Could you check a few things on this model? Use its own coordinates, in mm. Face numbers are marked on the shaded views. Coordinates: 2 decimals unless noted, no trailing zeros. Order: outer loops, then holes, each group sorted by start corner. A loop starts at its lowest first (then second) coordinate and runs counter-clockwise, first axis right, second up. Notation, with made-up numbers: M -22,29 L -3,29 A32 cw -3,65 Z; hole C 65,-39.75 d1. An arc over 180 degrees is marked long. Put each result on its own line as item: value. Start each with the question number.
Autodesk Inventor part; units mm, degrees
ref_plane "YZ Plane" through (0, 0, 0) normal (1, 0, 0) x (0, 1, 0)
ref_plane "XZ Plane" through (0, 0, 0) normal (0, 1, 0) x (-1, 0, 0)
ref_plane "XY Plane" through (0, 0, 0) normal (0, 0, 1) x (1, 0, 0)
sketch "Sketch1" plane through (0, 0, 0) normal (0, 0, 1) x (1, 0, 0)
  line L0 (4, 19.1204) -> (4, 20)
  line L1 (4, 20) -> (0, 20)
  line L2 (0, 20) -> (0, 16.5676)
  line L3 (0, 16.5676) -> (3.0669, 16.5676)
  line L4 (3.0669, 16.5676) -> (4.4257, 16)
  line L5 (4.4257, 16) -> (6.2458, 16)
  line L6 (6.2458, 16) -> (7, 16.7884)
  line L7 (7, 16.7884) -> (4, 19.1204)
  line L8 (0, 0) -> (20.4487, 0)
  dimension "d0" = 84.13
  dimension "d1" = 133.729
  dimension "d2" = 111.058
  dimension "d3" = 4
  dimension "d4" = 0.5675
  dimension "d5" = 4
  dimension "d6" = 0.7884
  dimension "d7" = 3
  dimension "d8" = 1.7197
  dimension "d9" = 32
revolve "Revolution1" add sketch "Sketch1" angle 360 about axis through (0, 0, 0) along (1, 0, 0)
properties part number "3136 7009 55" material "Nylon 6/6"
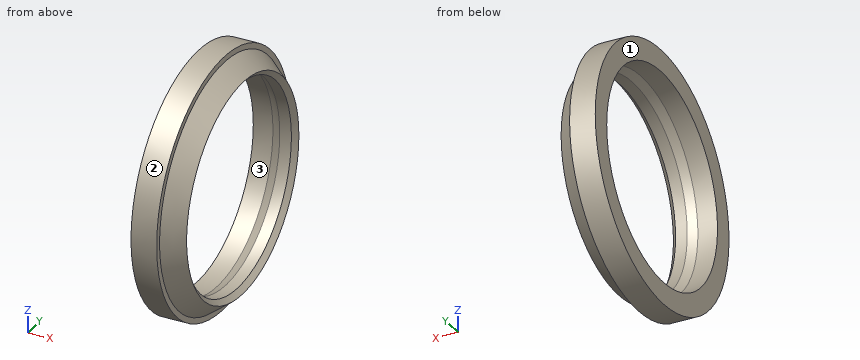
Item 1: For pin 1 Ø1.5 at (x, y) = (4.5, -5) entering from +Z; pin 2 Ø1.5 at (x, y) = (3.5, 9) entering from +Z; pin 3 Ø3 at (x, y) = (4.5, -13.5) entering from +Z, each with a flat end and sliding along its axis, tell me the tip position at first contact or that it passes through.
Item 2: If we mould it in two halves opening along Z, with no side actions, what happens to the marked faces 1, 2 and 3? For each: released by +Z, released by -Z, zero draft, split by the parting line, or undercut.
Item 3: If we section it at A-A on z = 0: Write out the boundary of the cut face in (x, y).
Item 4: I need wall thicknesses on probe 1 along Z at (x, y) = (1.7, 0); probe 2 along Y at (x, z) = (5.25, -2.5); probe 3 along Y at (x, z) = (1.5, -15). Which ranges of each line are inside material? Lowest first, please.
Item 5: If we section it at C-C on x = 1.25: Write out the boundary of the cut face in (y, z).
Geometry check:
1. pin 1: stops at z = 19.5
1. pin 2: stops at z = 18.22
1. pin 3: stops at z = 15.94
2. face 1: zero draft
2. face 2: split by the parting line
2. face 3: undercut
3. outline: M 0,-20 L 4,-20 L 4,-19.12 L 7,-16.79 L 6.25,-16 L 4.43,-16 L 3.07,-16.57 L 0,-16.57 Z; M 0,16.57 L 3.07,16.57 L 4.43,16 L 6.25,16 L 7,16.79 L 4,19.12 L 4,20 L 0,20 Z
4. probe 1: z = -20 to -16.57, 16.57 to 20
4. probe 2: y = -17.98 to -15.8, 15.8 to 17.98
4. probe 3: y = -13.23 to -7.03, 7.03 to 13.23
5. outline: C 0,0 d40; hole C 0,0 d33.14
